```python
from build123d import *
from build123d import SkipClean  # not in build123d's __all__

# Parameters (mm, degrees)
F1_DEPTH = 100
F3_DEPTH = 3
F4_DEPTH = 3
F6_DEPTH = 3
F7_R     = 10.25
F8_DEPTH = 3


# Not quite as in the source:
# - a feature names something its author has since deleted; it is built from what else it names


with BuildPart() as f1:
    # F0 (on Front) → F1 (new body)
    with BuildSketch(Plane.XZ):
        with BuildLine():
            Line((-44, 20.8545142158), (0, 20.8545142158))
            Line((0, 20.8545142158), (0, 23.8545142158))
            Line((0, 23.8545142158), (-44, 23.8545142158))
            ThreePointArc((-44, 23.8545142158), (-48.2426406871, 22.0971549029), (-50, 17.8545142158))
            Line((-50, 17.8545142158), (-50, -26.1454857842))
            Line((-50, -26.1454857842), (-47, -26.1454857842))
            Line((-47, -26.1454857842), (-47, 17.8545142158))
            ThreePointArc((-47, 17.8545142158), (-46.1213203436, 19.9758345594), (-44, 20.8545142158))
        make_face()
        with BuildLine():
            Line((0, 23.8545142158), (0, 20.8545142158))
            Line((0, 20.8545142158), (44, 20.8545142158))
            ThreePointArc((44, 20.8545142158), (46.1213203436, 19.9758345594), (47, 17.8545142158))
            Line((47, 17.8545142158), (47, -26.1454857842))
            Line((47, -26.1454857842), (50, -26.1454857842))
            Line((50, -26.1454857842), (50, 17.8545142158))
            ThreePointArc((50, 17.8545142158), (48.2426406871, 22.0971549029), (44, 23.8545142158))
            Line((44, 23.8545142158), (0, 23.8545142158))
        make_face()
    extrude(amount=F1_DEPTH)

    # F2 (on face) → F3 (cut)
    with BuildSketch(Plane(origin=(-50, 0, 0), x_dir=(0, -1, 0), z_dir=(-1, 0, 0))):
        with BuildLine():
            Line((39.75, -26.1454857842), (60.25, -26.1454857842))
            ThreePointArc((60.25, -26.1454857842), (50, -15.8954857842), (39.75, -26.1454857842))
        make_face()
    extrude(amount=-F3_DEPTH, mode=Mode.SUBTRACT)

    # F2 (on face) → F4 (join)
    with BuildSketch(Plane(origin=(-50, 0, 0), x_dir=(0, -1, 0), z_dir=(-1, 0, 0))):
        with BuildLine():
            Line((70, -26.1454857842), (60.25, -26.1454857842))
            ThreePointArc((60.25, -26.1454857842), (50, -36.3954857842), (39.75, -26.1454857842))
            Line((39.75, -26.1454857842), (30, -26.1454857842))
            Line((30, -26.1454857842), (30, -40.1454857842))
            ThreePointArc((30, -40.1454857842), (31.7573593129, -44.3881264713), (36, -46.1454857842))
            Line((36, -46.1454857842), (64, -46.1454857842))
            ThreePointArc((64, -46.1454857842), (68.2426406871, -44.3881264713), (70, -40.1454857842))
            Line((70, -40.1454857842), (70, -26.1454857842))
        make_face()
    with SkipClean():  # cleaning this boolean's faces spoils the solid; the shape is the same uncleaned
        extrude(amount=-F4_DEPTH)

    # F5 (on face) → F6 (join)
    with BuildSketch(Plane.YZ.offset(50)):
        with BuildLine():
            Line((-30, -26.1454857842), (-70, -26.1454857842))
            Line((-70, -26.1454857842), (-70, -40.1454857842))
            ThreePointArc((-70, -40.1454857842), (-68.2426406871, -44.3881264713), (-64, -46.1454857842))
            Line((-64, -46.1454857842), (-36, -46.1454857842))
            ThreePointArc((-36, -46.1454857842), (-31.7573593129, -44.3881264713), (-30, -40.1454857842))
            Line((-30, -40.1454857842), (-30, -26.1454857842))
        make_face()
    extrude(amount=-F6_DEPTH)

    # F7 (on face) → F8 (cut)
    with BuildSketch(Plane.YZ.offset(50)):
        with Locations((-50, -26.1454857842)):
            Circle(F7_R)
    extrude(amount=-F8_DEPTH, mode=Mode.SUBTRACT)


solid = f1.part
```
CAD build for the part. Positions are in the model's coordinates, mm. A direction names the side the tool comes from. Coordinates: 2 decimals unless noted, no trailing zeros. Write each loop counter-clockwise with the first axis right and the second up, starting at its lowest first coordinate (ties: lowest second). Pieces come first, ordered by that corner, then holes.
(1) Cut at A-A, the plane z = 9. List the corners of the cut face in (x, y), and give its area (3 significant figures).
(2) Flat gauge pins, fed straight in: pin 1 (1.5 mm diameter, centred on x = -49, y = -15.5, fed in from -Z); pin 2 (16.5 mm diameter, centred on y = -50, z = -26.15, fed in from -X); pin 3 (2.5 mm diameter, centred on x = 48, z = -34.5, fed in from -Y); pin 4 (1 mm diameter, centred on x = -24.5, y = -49, fed in from -Z). Where does each tip first touch, or does it go through?
(3) Cut at B-B, the plane y = -50. List the corners of the cut face in (x, z).
(4) 3-axis set-ups, long thin cutter, end or side, ignore diameter. For faces 4 (the face through (50, -49, -7)), 5 (the face through (49, -50, -46.145)), 6 (the face through (-49, -15, -26.145)), 7 (the face through (49, -70, -33)), 8 (the face through (46.098, -49.3, 19.999)): which of +Z, -Z, +X, -X, +Y, -Y reach the whole face in a straight line?
(5) Cut at D-D, the plane y = -12.5. List the corners of the cut face in (x, z).
(6) Drill centre lines: probe 1 along X at (y, z) = (-20.5, 8); probe 2 along Z at (x, y) = (-48, -50); probe 3 along Z at (x, y) = (-35, -17.5). Where is each one in solid material? Low to high.
(7) Cut at C-C, the plane z = -33. List the corners of the cut face in (x, y).
(8) Two-plate mould, pull along Y, no slides. Class faces 1 (the face through (-48.52, -59.78, -29.22)), 2 (the face through (48, -85, -26.145)), 3 (the face through (48.52, -68.29, -44.34)): +Y half, -Y half, draft (parallel to the pull), parting line (faces both ways), or undercut.
Geometry says:
1. outline: (-50, -100) - (-47, -100) - (-47, 0) - (-50, 0) - close; (47, -100) - (50, -100) - (50, 0) - (47, 0) - close
1. area: 600 mm2
2. pin 1: stops at z = -26.15
2. pin 2: passes through
2. pin 3: stops at y = -70
2. pin 4: stops at z = 20.85
3. outline: (-50, -46.15) - (-47, -46.15) - (-47, -36.4) - (-50, -36.4) - close; (-50, -15.9) - (-47, -15.9) - (-47, 17.85) arc R3 cw to (-44, 20.85) - (44, 20.85) arc R3 cw to (47, 17.85) - (47, -15.9) - (50, -15.9) - (50, 17.85) arc R6 ccw to (44, 23.85) - (-44, 23.85) arc R6 ccw to (-50, 17.85) - close; (47, -46.15) - (50, -46.15) - (50, -36.4) - (47, -36.4) - close
4. face 4: +Z, -Z, +X, +Y, -Y
4. face 5: -Z, +X, -X, +Y, -Y
4. face 6: -Z, +X, -X, +Y
4. face 7: -Z, +X, -X, -Y
4. face 8: -Z, +Y, -Y
5. outline: (-50, -26.15) - (-47, -26.15) - (-47, 17.85) arc R3 cw to (-44, 20.85) - (44, 20.85) arc R3 cw to (47, 17.85) - (47, -26.15) - (50, -26.15) - (50, 17.85) arc R6 ccw to (44, 23.85) - (-44, 23.85) arc R6 ccw to (-50, 17.85) - close
6. probe 1: x = -50 to -47, 47 to 50
6. probe 2: z = -46.15 to -36.4, -15.9 to 22.33
6. probe 3: z = 20.85 to 23.85
7. outline: (-50, -70) - (-47, -70) - (-47, -57.62) - (-50, -57.62) - close; (-50, -42.38) - (-47, -42.38) - (-47, -30) - (-50, -30) - close; (47, -70) - (50, -70) - (50, -57.62) - (47, -57.62) - close; (47, -42.38) - (50, -42.38) - (50, -30) - (47, -30) - close
8. face 1: undercut
8. face 2: draft
8. face 3: -Y half
